Source: three-view drawing plus pictorial views. Frame: mm from the lowest corner of the part. Round coordinates to 2 decimals unless told otherwise and drop trailing zeros. Loops run counter-clockwise (first coordinate to the right, second up) from the corner with the lowest first, then second, coordinate; pieces in that order, holes last. Notation, with made-up numbers: (70, 10) -> (99, 10) arc R18 ccw to (99, 27) -> close; hole circle Ø6 at (1.5, -3.5). An arc over 180 degrees is marked (long way). Return JSON: item names as keys, results as strings. Group by question number.
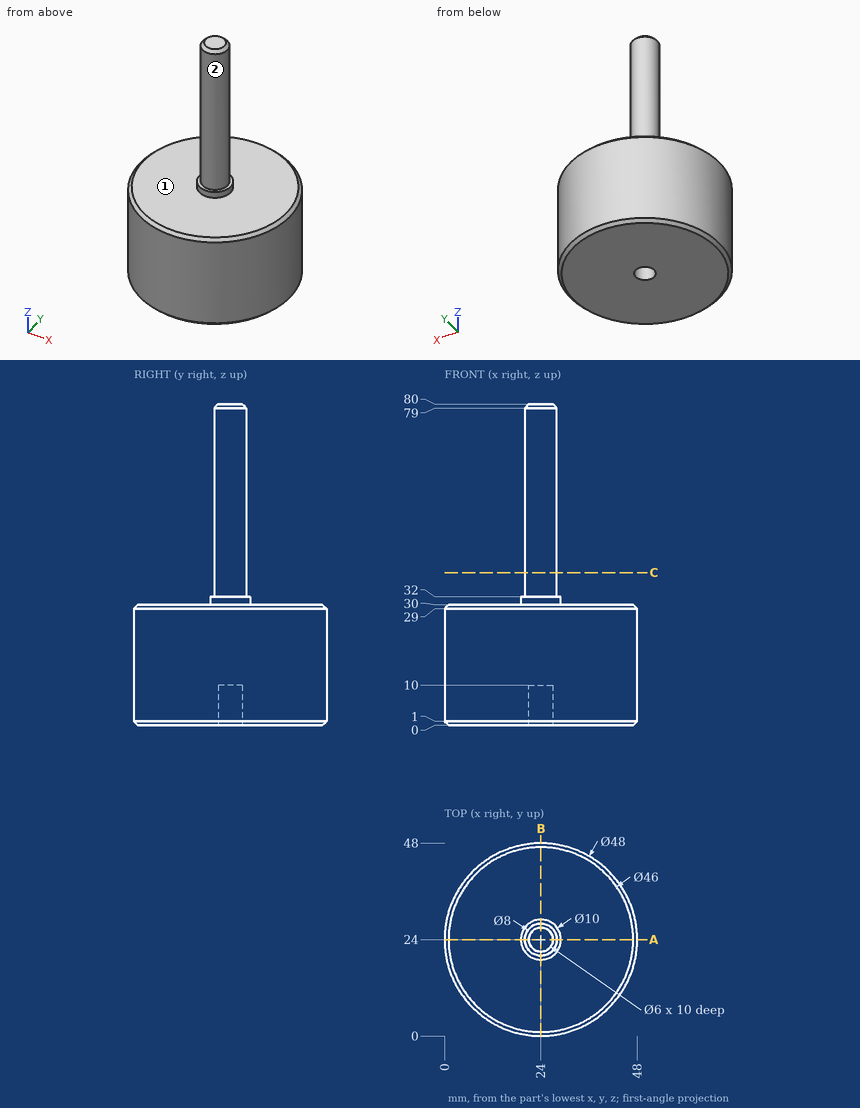
(1) Mould query, pull axis Y, two halves, no side actions, for the marked faces 1 and 2. Classes: released by +Y, released by -Y, zero draft, split by the parting line, or undercut.
(2) Ray query, line 1 (Y direction, x = 24, z = 5); line 2 (Z direction, x = 21.5, y = 31); line 3 (X direction, y = 24, z = 73). Return the intervals inside material, ascending.
(3) Pin query (flat end, axial travel): pin 1 (10 mm diameter, centred on x = 37.5, z = 34.5, fed in from +Y); pin 2 (4 mm diameter, centred on x = 22.5, z = 39.5, fed in from +Y); pin 3 (4 mm diameter, centred on y = 9.5, z = 17, fed in from -X); pin 4 (6 mm diameter, centred on x = 32.5, z = 60, fed in from +Y). Return the tip coordinate at first contact, or that it passes through.
(4) Cut plane A-A (y = 24). Return loops of the section in (x, z), and give its area (3 significant figures).
(5) Cut plane C-C (z = 38). Return loops of the section in (x, y).
Answers follow:
{
 "1": {"face 1": "zero draft", "face 2": "split by the parting line"},
 "2": {"line 1": "0 to 21, 27 to 48", "line 2": "0 to 30", "line 3": "20 to 28"},
 "3": {"pin 1": "y = 44.02", "pin 2": "y = 28", "pin 3": "x = 3.51", "pin 4": "through"},
 "4": {"outline": "(0, 1) -> (1, 0) -> (21, 0) -> (21, 10) -> (27, 10) -> (27, 0) -> (47, 0) -> (48, 1) -> (48, 29) -> (47, 30) -> (29, 30) -> (29, 32) -> (28, 32) -> (28, 79) -> (27, 80) -> (21, 80) -> (20, 79) -> (20, 32) -> (19, 32) -> (19, 30) -> (1, 30) -> (0, 29) -> close", "area": "1,780 mm^2"},
 "5": {"outline": "circle Ø8 at (24, 24)"}
}
